For this review, take the finished solid that the model builds, in its own axes (mm). Face numbers are marked on the shaded views. A direction names the side the tool comes from. Give positions to 0.01 mm unless a question says otherwise; leave off trailing zeros. Write each loop counter-clockwise with the first axis right and the second up, starting at its lowest first coordinate (ties: lowest second). Pieces come first, ordered by that corner, then holes.
Q1. Mouldability with a two-part tool opening along X and no side actions: class the marked faces 1, 2, 3 and 4 as released by +X, released by -X, zero draft, split by the parting line, or undercut.
Q2. We need section B-B (z = -10.5). Write out the cut boundary in (x, y).
Q3. We need section C-C (y = 9). Write out the cut boundary in (x, z).
Q4. For line 1 (Z direction, x = -21, y = 31.5); line 2 (X direction, y = 7, z = 13), list the stretches that pass through material, from the lowest coordinate up.
Q5. We need section A-A (x = 43). Write out the cut boundary in (y, z), then the cut area to 3 significant figures.
Q6. Insertion check: P1, Ø1.6, axis at y = 6, z = 30, coming from the +X side; P2, Ø0.8, axis at y = 7, z = 30.5, coming from the -X side; P3, Ø8, axis at x = 3.5, z = 25.5, coming from the +Y side. Each pin has a flat end and moves straight along its axis. Give the tip position at first contact, or say it passes through.
Q7. Machinability: for the marked faces 5 and 6, which of the approach directions +Z, -Z, +X, -X, +Y, -Y give a long, thin tool a straight path to every point of the face, cutting with its end or side? Answer none if there is none.
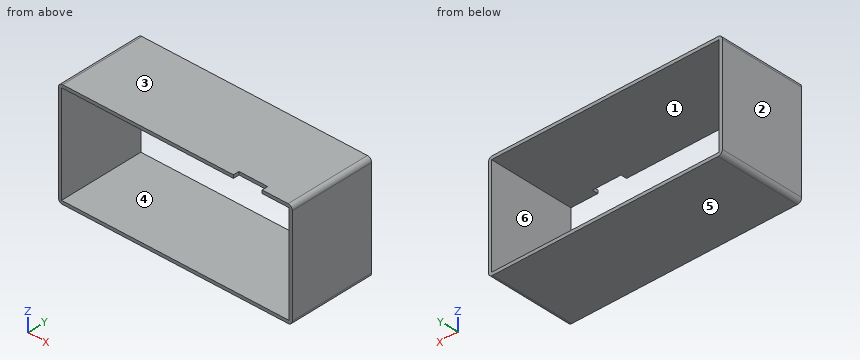
```python
from build123d import *

# Parameters (mm, degrees)
STOCK_FULL_START               = 5
STOCK_FULL_SHAPE_1_OUTLINE_W   = 110
STOCK_FULL_SHAPE_1_OUTLINE_H   = 50
STOCK_FULL_SHAPE_1_OUTLINE_W_2 = 107
STOCK_FULL_SHAPE_1_OUTLINE_H_2 = 47
STOCK_FULL_SHAPE_1_DEPTH       = 40
FILLET1_R                      = 2
SKETCH3_W                      = 13.5
SKETCH3_H                      = 1.5
CUT_EXTRUDE1_DEPTH             = 2.8


# Read off the part's stored shape, not the designer's step: Stock-full shape-1
with BuildPart() as part:
    # Stock-full shape-1 outline → Stock-full shape-1 (new body)
    with BuildSketch(Plane(origin=(0, 0, 0), x_dir=(1, 0, 0), z_dir=(0, 1, 0)).offset(STOCK_FULL_START)):
        with Locations((14.090909091, -5.886363636)):
            Rectangle(STOCK_FULL_SHAPE_1_OUTLINE_W, STOCK_FULL_SHAPE_1_OUTLINE_H)
        with Locations((14.090909091, -5.886363636)):
            Rectangle(STOCK_FULL_SHAPE_1_OUTLINE_W_2, STOCK_FULL_SHAPE_1_OUTLINE_H_2, mode=Mode.SUBTRACT)
    extrude(amount=STOCK_FULL_SHAPE_1_DEPTH)

    # Fillet1
    fillet1_edges = [part.edges().sort_by_distance(p)[0] for p in [
        (-40.909090909, 25, -19.113636364),
        (69.090909091, 25, -19.113636364),
        (69.090909091, 25, 30.886363636),
        (-40.909090909, 25, 30.886363636),
    ]]
    fillet(fillet1_edges, radius=FILLET1_R)

    # Sketch3 → Cut-Extrude1 (cut)
    with BuildSketch(Plane.XZ.offset(-5)):
        with Locations((48.140909091, 30.136363636)):
            Rectangle(SKETCH3_W, SKETCH3_H)
    extrude(amount=-CUT_EXTRUDE1_DEPTH, mode=Mode.SUBTRACT)


solid = part.part
```
Computed:
1. face 1: undercut
1. face 2: released by -X
1. face 3: zero draft
1. face 4: undercut
2. outline: (-40.91, 5) - (-39.41, 5) - (-39.41, 45) - (-40.91, 45) - close; (67.59, 5) - (69.09, 5) - (69.09, 45) - (67.59, 45) - close
3. outline: (-40.91, -17.11) arc R2 ccw to (-38.91, -19.11) - (67.09, -19.11) arc R2 ccw to (69.09, -17.11) - (69.09, 28.89) arc R2 ccw to (67.09, 30.89) - (-38.91, 30.89) arc R2 ccw to (-40.91, 28.89) - close; hole (-39.41, -17.61) - (67.59, -17.61) - (67.59, 29.39) - (-39.41, 29.39) - close
4. line 1: z = -19.11 to -17.61, 29.39 to 30.89
4. line 2: x = -40.91 to -39.41, 67.59 to 69.09
5. outline: (5, -19.11) - (45, -19.11) - (45, -17.61) - (5, -17.61) - close; (7.8, 29.39) - (45, 29.39) - (45, 30.89) - (7.8, 30.89) - close
5. area: 116 mm2
6. P1: stops at x = 69.07
6. P2: stops at x = -40.5
6. P3: stops at y = 45
7. face 5: -Z, +X, -X, +Y, -Y
7. face 6: +Y, -Y
